from build123d import *

# Parameters (mm, degrees)
SKETCH2_R           = 16.7005
SKETCH2_R_2         = 13.3223
BOSS_EXTRUDE1_DEPTH = 76.2


with BuildPart() as part:
    # Sketch2 → Boss-Extrude1 (new body)
    with BuildSketch(Plane.XY):
        with Locations(Location((0, 0, 0), (0, 0, 180))):
            Circle(SKETCH2_R)
        with Locations(Location((0, 0, 0), (0, 0, 180))):
            Circle(SKETCH2_R_2, mode=Mode.SUBTRACT)
    extrude(amount=BOSS_EXTRUDE1_DEPTH)

    # Sketch3 → Cut-Revolve2 (revolve, cut)
    with BuildSketch(Plane(origin=(0, 0, 0), x_dir=(0, 0, -1), z_dir=(1, 0, 0)), mode=Mode.PRIVATE) as cut_revolve2_sk:
        Polygon((0, 21.813584822), (-19.05, 21.813584822), (-19.05, 16.7005), (-19.05, 15.869250272), (0, 15.126208453), align=None)
        Polygon((-76.2, 15.126208453), (-76.2, 21.813584822), (-57.15, 21.813584822), (-57.15, 16.7005), (-57.15, 15.869250272), align=None)
    revolve(cut_revolve2_sk.sketch.rotate(Axis((0, 0, 38.1), (0, 0, 1)), 90), axis=Axis((0, 0, 38.1), (0, 0, 1)), mode=Mode.SUBTRACT)


solid = part.part
Input: part model. Units: mm. Frame: model coordinates. A direction names the side the tool comes from. Coordinates: 2 decimals unless noted, no trailing zeros. Loops run counter-clockwise (first coordinate to the right, second up) from the corner with the lowest first, then second, coordinate; pieces in that order, holes last.
(1) Section A-A on y = 0. Return the cut outline in (x, z), then the cut area to 3 significant figures.
(2) Section C-C on z = 32. Return the cut outline in (x, y).
(3) Set-up query: faces 1 (the face through (-15, 6, 19.05)), 2 (the face through (-5.5, 12.3, 76.2)). Return all of +Z, -Z, +X, -X, +Y, -Y with unobstructed straight access to the full face (end or side cutting, diameter ignored); none if empty.
(4) Section D-D on z = 63. Return the cut outline in (x, y).
(5) Material intervals for probe 1 along Y at (x, z) = (0, 37); probe 2 along Y at (x, z) = (5, 32); probe 3 along X at (y, z) = (-1, 19), sorted ascending.
(6) Pull-direction query (Y, two-part tool) for faces 3 (the face through (-12.707, -4.002, 37.567)), 4 (the face through (-15.93, -5.02, 37.83)), 5 (the face through (15, 6, 57.15)); classes: released by +Y, released by -Y, zero draft, split by the parting line, or undercut.
(7) First-contact query: pin 1 Ø1.5 at (x, z) = (-6.5, 43) entering from -Y; pin 2 Ø5 at (x, z) = (11.5, 42.5) entering from +Y. Flat tips, straight axial feed; report the tip coordinate or a pass-through.
Data:
1. outline: (-16.7, 19.05) - (-15.87, 19.05) - (-15.13, 0) - (-13.32, 0) - (-13.32, 76.2) - (-15.13, 76.2) - (-15.87, 57.15) - (-16.7, 57.15) - close; (13.32, 0) - (15.13, 0) - (15.87, 19.05) - (16.7, 19.05) - (16.7, 57.15) - (15.87, 57.15) - (15.13, 76.2) - (13.32, 76.2) - close
1. area: 423 mm2
2. outline: circle Ø33.4 at (0, 0); hole circle Ø26.64 at (0, 0)
3. face 1: -Z
3. face 2: +Z, +X, -X, +Y, -Y
4. outline: circle Ø31.28 at (0, 0); hole circle Ø26.64 at (0, 0)
5. probe 1: y = -16.7 to -13.32, 13.32 to 16.7
5. probe 2: y = -15.93 to -12.35, 12.35 to 15.93
5. probe 3: x = -15.84 to -13.28, 13.28 to 15.84
6. face 3: undercut
6. face 4: split by the parting line
6. face 5: zero draft
7. pin 1: stops at y = -15.68
7. pin 2: stops at y = 14.07
